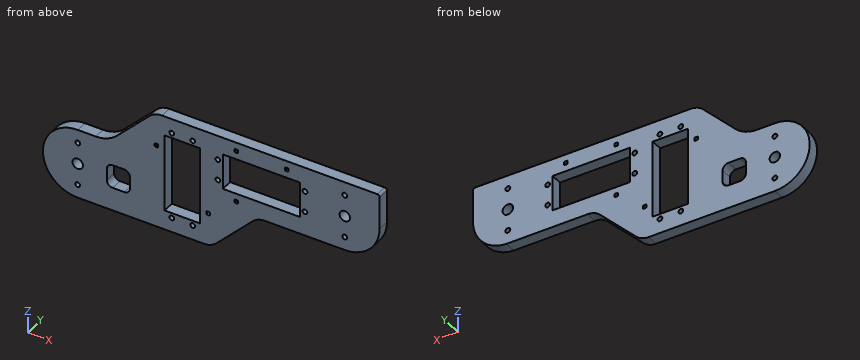
Autodesk Fusion 360 part; units mm, degrees
sketch "outline" plane through (0, 0, 0) normal (0, 1, 0) x (-1, 0, 0)
  circle A0 centre (115, -20) radius 4.5
  circle A1 centre (-115, 20) radius 4.5
  circle A2 centre (115, -38.5) radius 2.1
  circle A3 centre (115, -1.5) radius 2.1
  line L0 (115, 10) -> (99.5972, 10)
  line L1 (81.0587, 17.6789) -> (53.131, 45.6066)
  line L2 (42.5244, 50) -> (-143, 50)
  line L3 (115, -50) -> (20.0095, -50)
  arc A4 (81.0587, 17.6789) -> (99.5972, 10) centre (99.5972, 36.2173) ccw
  arc A5 (53.131, 45.6066) -> (42.5244, 50) centre (42.5244, 35) ccw
  circle A6 centre (-115, 38.5) radius 2.1
  circle A7 centre (-115, 1.5) radius 2.1
  line L4 (-116.33, -10) -> (-46.2132, -10)
  line L5 (-145, 48) -> (-145, 19.9705)
  arc A8 (-145, 19.9705) -> (-116.33, -10) centre (-115, 19.9705) ccw
  line L6 (6.2132, -50) -> (20.0095, -50)
  line L7 (-35.6066, -14.3934) -> (-4.3934, -45.6066)
  arc A9 (115, -50) -> (115, 10) centre (115, -20) ccw
  line L8 (40.268, -33.25) -> (40.268, 33.25)
  line L9 (9.768, -33.25) -> (40.268, -33.25)
  line L10 (40.268, 33.25) -> (9.768, 33.25)
  line L11 (9.768, 33.25) -> (9.768, -33.25)
  circle A10 centre (16.018, 37.5) radius 2.05
  circle A11 centre (16.018, -37.5) radius 2.05
  circle A12 centre (34.018, -37.5) radius 2.05
  circle A13 centre (34.018, 37.5) radius 2.05
  line L12 (-76.45, 4.75) -> (-9.95, 4.75)
  line L13 (-76.45, 35.25) -> (-76.45, 4.75)
  line L14 (-9.95, 4.75) -> (-9.95, 35.25)
  line L15 (-9.95, 35.25) -> (-76.45, 35.25)
  circle A14 centre (-5.7, 29) radius 2.05
  circle A15 centre (-80.7, 29) radius 2.05
  circle A16 centre (-80.7, 11) radius 2.05
  circle A17 centre (-5.7, 11) radius 2.05
  arc A18 (-4.3934, -45.6066) -> (6.2132, -50) centre (6.2132, -35) ccw
  arc A19 (-35.6066, -14.3934) -> (-46.2132, -10) centre (-46.2132, -25) ccw
  line L16 (85, -30) -> (75, -30)
  line L17 (70, -25) -> (70, -15)
  line L18 (75, -10) -> (85, -10)
  line L19 (90, -15) -> (90, -25)
  arc A20 (85, -30) -> (90, -25) centre (85, -25) ccw
  arc A21 (90, -15) -> (85, -10) centre (85, -15) ccw
  arc A22 (75, -10) -> (70, -15) centre (75, -15) ccw
  arc A23 (70, -25) -> (75, -30) centre (75, -25) ccw
  arc A24 (-143, 50) -> (-145, 48) centre (-143, 48) ccw
  dimension "d1" = 9
  dimension "d15" = 4.2
  dimension "d16" = 18.5
  dimension "d17" = 37
  dimension "d24" = 135
  dimension "d25" = 60
  dimension "d36" = 30
  dimension "d40" = 15
  dimension "d86" = 4.2
  dimension "d87" = 4.2
  dimension "d88" = 37
  dimension "d89" = 18.5
  dimension "d98" = 100
  dimension "d99" = 115
  dimension "d100" = 50
  dimension "d105" = 30
  dimension "d109" = 75
  dimension "d110" = 230
  dimension "d111" = 30
  dimension "d112" = 30
  dimension "d157" = 15.25
  dimension "d158" = 15.25
  dimension "d159" = 33.25
  dimension "d160" = 33.25
  dimension "d161" = 4.1
  dimension "d162" = 18
  dimension "d163" = 75
  dimension "d167" = 15.25
  dimension "d168" = 9
  dimension "d169" = 37.5
  dimension "d170" = 18
  dimension "d172" = 15.25
  dimension "d173" = 15.25
  dimension "d174" = 33.25
  dimension "d175" = 33.25
  dimension "d176" = 4.1
  dimension "d177" = 18
  dimension "d178" = 75
  dimension "d181" = 18.2
  dimension "d182" = 15.25
  dimension "d183" = 37.5
  dimension "d184" = 9
  dimension "d185" = 90
  dimension "d228" = 15
  dimension "d229" = 15
  dimension "d230" = 5
  dimension "d231" = 20
  dimension "d232" = 25
  dimension "d233" = 135
  dimension "d234" = 2
  dimension "d270" = 18.2
  dimension "d271" = 90
extrude "Extrusion2" add sketch "outline" along normal blind 10
sketch "Skizze3" plane through (0, 10, 0) normal (0, 1, 0) x (-1, 0, 0)
  circle A0 centre (16.018, 37.5) radius 2.05
  circle A1 centre (16.018, -37.5) radius 2.05
  circle A2 centre (34.018, -37.5) radius 2.05
  circle A3 centre (34.018, 37.5) radius 2.05
  circle A4 centre (-115, 1.5) radius 2.1
  line L0 (9.768, -33.25) -> (9.768, 33.25)
  line L1 (9.768, 33.25) -> (40.268, 33.25)
  line L2 (40.268, 33.25) -> (40.268, -33.25)
  line L3 (40.268, -33.25) -> (9.768, -33.25)
  circle A5 centre (-115, 38.5) radius 2.1
  circle A6 centre (115, -1.5) radius 2.1
  circle A7 centre (115, -38.5) radius 2.1
  circle A8 centre (-115, 20) radius 4.5
  circle A9 centre (115, -20) radius 4.5
  circle A10 centre (-80.7, 11) radius 2.05
  circle A11 centre (-5.7, 11) radius 2.05
  circle A12 centre (-80.7, 29) radius 2.05
  circle A13 centre (-5.7, 29) radius 2.05
  line L4 (-76.45, 35.25) -> (-9.95, 35.25)
  line L5 (-9.95, 35.25) -> (-9.95, 4.75)
  line L6 (-9.95, 4.75) -> (-76.45, 4.75)
  line L7 (-76.45, 4.75) -> (-76.45, 35.25)
  line L8 (81.0587, 17.6789) -> (53.131, 45.6066)
  arc A14 (53.131, 45.6066) -> (42.5244, 50) centre (42.5244, 35) ccw
  line L9 (42.5244, 50) -> (-143, 50)
  line L10 (-145, 48) -> (-145, 19.9705)
  arc A15 (-145, 19.9705) -> (-116.33, -10) centre (-115, 19.9705) ccw
  line L11 (-116.33, -10) -> (-46.2132, -10)
  line L12 (-35.6066, -14.3934) -> (-4.3934, -45.6066)
  line L13 (6.2132, -50) -> (115, -50)
  arc A16 (115, -50) -> (115, 10) centre (115, -20) ccw
  line L14 (115, 10) -> (99.5972, 10)
  arc A17 (81.0587, 17.6789) -> (99.5972, 10) centre (99.5972, 36.2173) ccw
  line L15 (6.2132, -50) -> (20.0095, -50)
  line L16 (115, -50) -> (20.0095, -50)
  line L17 (42.5244, 50) -> (-143, 50)
  arc A18 (-4.3934, -45.6066) -> (6.2132, -50) centre (6.2132, -35) ccw
  arc A19 (-35.6066, -14.3934) -> (-46.2132, -10) centre (-46.2132, -25) ccw
  arc A20 (75, -10) -> (70, -15) centre (75, -15) ccw
  line L18 (75, -10) -> (85, -10)
  arc A21 (90, -15) -> (85, -10) centre (85, -15) ccw
  line L19 (90, -15) -> (90, -25)
  arc A22 (85, -30) -> (90, -25) centre (85, -25) ccw
  line L20 (85, -30) -> (75, -30)
  arc A23 (70, -25) -> (75, -30) centre (75, -25) ccw
  line L21 (70, -25) -> (70, -15)
  arc A24 (-143, 50) -> (-145, 48) centre (-143, 48) ccw
  line L22 (48.268, 20.25) -> (46.268, 20.25)
  line L23 (45.768, 20.75) -> (45.768, 22.75)
  line L24 (46.268, 23.25) -> (48.268, 23.25)
  line L25 (48.768, 22.75) -> (48.768, 20.75)
  arc A25 (48.768, 22.75) -> (48.268, 23.25) centre (48.268, 22.75) ccw
  arc A26 (48.268, 20.25) -> (48.768, 20.75) centre (48.268, 20.75) ccw
  arc A27 (45.768, 20.75) -> (46.268, 20.25) centre (46.268, 20.75) ccw
  arc A28 (46.268, 23.25) -> (45.768, 22.75) centre (46.268, 22.75) ccw
  line L26 (1.268, -22.75) -> (1.268, -20.75)
  arc A29 (3.768, -23.25) -> (4.268, -22.75) centre (3.768, -22.75) ccw
  arc A30 (1.768, -20.25) -> (1.268, -20.75) centre (1.768, -20.75) ccw
  line L27 (1.768, -20.25) -> (3.768, -20.25)
  arc A31 (4.268, -20.75) -> (3.768, -20.25) centre (3.768, -20.75) ccw
  line L28 (4.268, -20.75) -> (4.268, -22.75)
  arc A32 (1.268, -22.75) -> (1.768, -23.25) centre (1.768, -22.75) ccw
  line L29 (3.768, -23.25) -> (1.768, -23.25)
  line L30 (-22.95, 41.5) -> (-22.95, 43.5)
  arc A33 (-20.45, 41) -> (-19.95, 41.5) centre (-20.45, 41.5) ccw
  arc A34 (-22.45, 44) -> (-22.95, 43.5) centre (-22.45, 43.5) ccw
  line L31 (-22.45, 44) -> (-20.45, 44)
  arc A35 (-19.95, 43.5) -> (-20.45, 44) centre (-20.45, 43.5) ccw
  line L32 (-19.95, 43.5) -> (-19.95, 41.5)
  arc A36 (-22.95, 41.5) -> (-22.45, 41) centre (-22.45, 41.5) ccw
  line L33 (-20.45, 41) -> (-22.45, 41)
  line L34 (-66.45, 41.5) -> (-66.45, 43.5)
  arc A37 (-63.95, 41) -> (-63.45, 41.5) centre (-63.95, 41.5) ccw
  arc A38 (-65.95, 44) -> (-66.45, 43.5) centre (-65.95, 43.5) ccw
  line L35 (-65.95, 44) -> (-63.95, 44)
  arc A39 (-63.45, 43.5) -> (-63.95, 44) centre (-63.95, 43.5) ccw
  line L36 (-63.45, 43.5) -> (-63.45, 41.5)
  arc A40 (-66.45, 41.5) -> (-65.95, 41) centre (-65.95, 41.5) ccw
  line L37 (-63.95, 41) -> (-65.95, 41)
  line L38 (-20.45, -3.75) -> (-22.45, -3.75)
  line L39 (-19.95, -1.25) -> (-19.95, -3.25)
  arc A41 (-20.45, -3.75) -> (-19.95, -3.25) centre (-20.45, -3.25) ccw
  arc A42 (-22.45, -0.75) -> (-22.95, -1.25) centre (-22.45, -1.25) ccw
  arc A43 (-22.95, -3.25) -> (-22.45, -3.75) centre (-22.45, -3.25) ccw
  line L40 (-22.95, -3.25) -> (-22.95, -1.25)
  line L41 (-22.45, -0.75) -> (-20.45, -0.75)
  arc A44 (-19.95, -1.25) -> (-20.45, -0.75) centre (-20.45, -1.25) ccw
  point P0 (-269.883, 0)
  dimension "d235" = 3
  dimension "d236" = 3
  dimension "d237" = 0.5
  dimension "d238" = 10
  dimension "d239" = 5.5
  dimension "d240" = 3
  dimension "d241" = 3
  dimension "d242" = 0.5
  dimension "d244" = 5.5
  dimension "d245" = 3
  dimension "d246" = 3
  dimension "d247" = 0.5
  dimension "d248" = 6
  dimension "d251" = 10
  dimension "d255" = 3
  dimension "d256" = 3
  dimension "d257" = 0.5
  dimension "d260" = 10
  dimension "d261" = 6
  dimension "d262" = 10
  dimension "d263" = 3
  dimension "d264" = 3
  dimension "d265" = 0.5
  dimension "d266" = 10
  dimension "d267" = 5.5
extrude "Extrusion5" cut sketch "Skizze3" against normal blind 10 contours L22 L23 L24 L25 A25 A26 A27 A28 | L26 A29 A30 L27 A31 L28 A32 L29 | L30 A33 A34 L31 A35 L32 A36 L33 | L34 A37 A38 L35 A39 L36 A40 L37 | L38 L39 A41 A42 A43 L40 L41 A44
equation "Belt_Diameter = 90 mm"
equation "d157 = 15 mm + tolerance"
equation "d158 = 15 mm + tolerance"
equation "d159 = 33 mm + tolerance"
equation "d160 = 33 mm + tolerance"
equation "d167 = 15 mm + tolerance"
equation "d172 = 15 mm + tolerance"
equation "d173 = 15 mm + tolerance"
equation "d174 = 33 mm + tolerance"
equation "d175 = 33 mm + tolerance"
equation "d182 = 15 mm + tolerance"
equation "tolerance = 0.25 mm"
Check sheet for the modelled part. Datum: model origin and axes. Units: mm. Round coordinates to 2 decimals unless told otherwise and drop trailing zeros. Loops run counter-clockwise (first coordinate to the right, second up) from the corner with the lowest first, then second, coordinate; pieces in that order, holes last. Notation, with made-up numbers: (-17, 60.5) -> (9, 60.5) arc R15 ccw to (9, 76.5) -> close; hole circle Ø11 at (-17.5, -31). An arc over 180 degrees is marked (long way). Answer in a Markdown table with one row per item.
Q1. Go/stop test with flat-tipped pins: P1, Ø1, axis at y = 5.5, z = 26.5, coming from the -X side; P2, Ø3.5, axis at x = -115, z = -1.5, coming from the -Y side; P3, Ø4, axis at x = 6.5, y = 4, coming from the -Z side; P4, Ø0.6, axis at y = 7, z = 42, coming from the -X side. Record where each tip stops, or that it passes through.
Data:
| item | result |
|---|---|
| P1 | stops at x = -72.74 |
| P2 | passes through |
| P3 | stops at z = -45.5 |
| P4 | stops at x = -57.04 |
Q2. Sectioned sample at A-A on x = -25. Enter the section's corners in (y, z).
Data:
| item | result |
|---|---|
| outline | (0, -50) -> (10, -50) -> (10, -33.25) -> (0, -33.25) -> close; (0, 33.25) -> (10, 33.25) -> (10, 50) -> (0, 50) -> close |
Q3. Sectioned sample at B-B on y = 3.25. Give the number of separate pieces and of enclosed holes in the cut face, then the cut area to 3 significant figures.
Data:
| item | result |
|---|---|
| separate pieces | 1 |
| enclosed holes | 22 |
| area | 15,600 mm^2 |
Q4. Sectioned sample at C-C on x = 103.5. Enter the section's corners in (y, z), then the cut area to 3 significant figures.
Data:
| item | result |
|---|---|
| outline | (0, -10) -> (10, -10) -> (10, 50) -> (0, 50) -> close |
| area | 600 mm^2 |
Q5. Thickness scan on L1, parallel to Z at x = 80.7, y = 5.5; L2, parallel to Z at x = -115, y = 7.5; L3, parallel to Z at x = 18, y = 5. Record the ranges inside material, lowest first.
Data:
| item | result |
|---|---|
| L1 | z = -10 to 8.95, 13.05 to 26.95, 31.05 to 50 |
| L2 | z = -50 to -40.6, -36.4 to -24.5, -15.5 to -3.6, 0.6 to 10 |
| L3 | z = -32 to 4.75, 35.25 to 50 |
